from build123d import *

# Parameters (mm, degrees)
F1_DEPTH = 25.4
F2_T     = -2.54


with BuildPart() as f1:
    # F0 (on Front) → F1 (new body)
    with BuildSketch(Plane.XZ):
        with BuildLine():
            Line((0, 38.503944), (0, 47.30061))
            ThreePointArc((0, 47.30061), (-33.446582, 33.446582), (-47.30061, 0))
            Line((-47.30061, 0), (-38.503944, 0))
            ThreePointArc((-38.503944, 0), (-27.2264, 27.2264), (0, 38.503944))
        make_face()
    extrude(amount=F1_DEPTH)

    # F2
    f2_openings = [f1.faces().sort_by_distance(p)[0] for p in [
        (0, -12.7, 42.902277),
    ]]
    offset(amount=F2_T, openings=f2_openings)


solid = f1.part
Geometry check sheet. Reference: the model listing, model coordinates, mm. A direction names the side the tool comes from. Give positions to 0.01 mm unless a question says otherwise; leave off trailing zeros. Write each loop counter-clockwise with the first axis right and the second up, starting at its lowest first coordinate (ties: lowest second). Pieces come first, ordered by that corner, then holes. Notation, with made-up numbers: M 86,-3 L 115,-3 A18 cw 115,19 Z; hole C 20.5,35.25 d7. An arc over 180 degrees is marked long. Answer as CSV lines item,"result". Start each with the question number.
Q1. Go/stop test with flat-tipped pins: pin 1 (3 mm diameter, centred on x = -6, y = -11.5, fed in from +Z); pin 2 (1 mm diameter, centred on x = -21, y = -16, fed in from +Z); pin 3 (1.5 mm diameter, centred on x = -19.5, y = -18.5, fed in from -Z). Record where each tip stops, or that it passes through.
Q2. Section check B-B, the plane z = 17. Record the cut outline in (x, y).
Q3. Section check A-A, the plane x = -39.5. Record the cut outline in (y, z).
Q4. Tool access check on faces 4 (the face through (-27.52, -12.52, 26.93)), 5 (the face through (-28.42, -12.56, 29.61)). Record the directions out of +Z, -Z, +X, -X, +Y, -Y that give a thin tool (end or side, any length) a straight path to the whole face; none if there is none.
Q5. Release check for a two-part mould opening along Y. For faces 1 (the face through (-29, -25.4, 27)), 2 (the face through (-43, -13, 2.54)), 3 (the face through (0, -13, 45)) record: pulls with the +Y half, pulls with the -Y half, needs draft (parallel to the pull), parting line crosses it, or undercut.
Q6. Material ranges on L1, parallel to Y at x = -36, z = 21; L2, parallel to Z at x = -15.5, y = -19.25; L3, parallel to X at y = -9.75, z = 17.5, recorded low to high.
Q7. Section check C-C, the plane y = -20. Record the cut outline in (x, z), then the cut area to 3 significant figures.
Geometry says:
1,pin 1,"z = 47.09"
1,pin 2,"z = 42.63"
1,pin 3,"z = 32.75"
2,outline,"M -44.14,-25.4 L -34.55,-25.4 L -34.55,0 L -44.14,0 Z; hole M -41.41,-22.86 L -37.36,-22.86 L -37.36,-2.54 L -41.41,-2.54 Z"
3,outline,"M -25.4,0 L 0,0 L 0,26.02 L -25.4,26.02 Z; hole M -22.86,11.15 L -2.54,11.15 L -2.54,21.05 L -22.86,21.05 Z"
4,face 4,"-Z, +X, +Y, -Y"
4,face 5,"none"
5,face 1,"pulls with the -Y half"
5,face 2,"undercut"
5,face 3,"needs draft"
6,L1,"-25.4 to -22.86, -2.54 to 0"
6,L2,"35.25 to 38, 41.99 to 44.69"
6,L3,"-43.94 to -41.2, -37.13 to -34.3"
7,outline,"M -47.3,0 L -38.5,0 A38.5 cw 0,38.5 L 0,41.04 A41.04 ccw -40.97,2.54 L -44.69,2.54 A44.76 cw 0,44.76 L 0,47.3 A47.3 ccw Z"
7,area,"352 mm^2"
